Verification items for the finished model (mm, model axes). Coordinates: 2 decimals unless noted, no trailing zeros. Loops run counter-clockwise (first coordinate to the right, second up) from the corner with the lowest first, then second, coordinate; pieces in that order, holes last. Notation, with made-up numbers: (23, -39) - (45, -39) arc R8 ccw to (45, -26) - close; hole circle Ø2 at (-8, 71.25). An arc over 180 degrees is marked (long way). One line per item, written item: value. Start each with the question number.
(1) Section check C-C (x = 388). Record the boundary of the cut face in (y, z) (3 decimals).
(2) Gauge pin test, flat ends, axial feed: P1, Ø12, axis at y = -497, z = 12.5, coming from the -X side; P2, Ø8, axis at y = -641.5, z = 17.5, coming from the -X side. Record the tip position at first contact, or that the pin passes through.
(3) Draft check along Z on faces 1 (the face through (-15, -110, 28.575)), 2 (the face through (-15.65, -882.386, 14.087)), 3 (the face through (-15, -110, 0)). Enter one of: +Z half, -Z half, draft (parallel to the pull), parting line (faces both ways), or undercut.
(4) Section check B-B (x = 73.5). Record the boundary of the cut face in (y, z) (3 decimals), plus the area to 3 significant figures.
(5) Section check D-D (x = -331.5). Record the boundary of the cut face in (y, z) (3 decimals).
(6) Section check A-A (z = 5.5). Record the boundary of the cut face in (x, y).
(7) Thickness scan on probe 1 along Y at (x, z) = (0, 12.25); probe 2 along X at (y, z) = (-188.5, 19.5); probe 3 along Y at (x, z) = (-6, 17.5). Record the ranges inside material, lowest first. Write a range as [from, to].
```python
from build123d import *

# Parameters (mm, degrees)
F1_DEPTH = 28.575


# Not quite as in the source:
# - a feature names something its author has since deleted; it is built from what else it names


with BuildPart() as f1:
    # F0 (on Top) → F1 (new body)
    with BuildSketch(Plane.XY):
        with BuildLine():
            ThreePointArc((-1037.5478672986, -524.8695620945), (-548.7202955818, -790.5538516378), (0, -882.4590952158))
            ThreePointArc((0, -882.4590952158), (548.7202955818, -790.5538516378), (1037.5478672986, -524.8695620945))
            ThreePointArc((1037.5478672986, -524.8695620945), (1059.0976915237, -498.2343056164), (1066.8, -464.8500839552))
            Line((1066.8, -464.8500839552), (1066.8, -44.2590952158))
            Line((1066.8, -44.2590952158), (1066.8, 641.5409047842))
            Line((1066.8, 641.5409047842), (-1066.8, 641.5409047842))
            Line((-1066.8, 641.5409047842), (-1066.8, -44.2590952158))
            Line((-1066.8, -44.2590952158), (-1066.8, -464.8500839552))
            ThreePointArc((-1066.8, -464.8500839552), (-1059.0976915237, -498.2343056164), (-1037.5478672986, -524.8695620945))
        make_face()
        Polygon((-139.7, -165.1), (0, -165.1), (139.7, -165.1), (139.7, -292.1), (0, -292.1), (-139.7, -292.1), align=None, mode=Mode.SUBTRACT)
        with BuildLine():
            ThreePointArc((0, -25.4), (-17.9605122421, 17.9605122421), (25.4, 0))
            ThreePointArc((25.4, 0), (17.9605122421, -17.9605122421), (0, -25.4))
        make_face(mode=Mode.SUBTRACT)
    extrude(amount=F1_DEPTH)


solid = f1.part
```
Responses:
1. outline: (-837.152, 0) - (641.541, 0) - (641.541, 28.575) - (-837.152, 28.575) - close
2. P1: stops at x = -1062.17
2. P2: stops at x = -874.66
3. face 1: +Z half
3. face 2: draft
3. face 3: -Z half
4. outline: (-880.854, 0) - (-292.1, 0) - (-292.1, 28.575) - (-880.854, 28.575) - close; (-165.1, 0) - (641.541, 0) - (641.541, 28.575) - (-165.1, 28.575) - close
4. area: 39,900 mm²
5. outline: (-849.509, 0) - (641.541, 0) - (641.541, 28.575) - (-849.509, 28.575) - close
6. outline: (-1066.8, -464.85) arc R76.2 ccw to (-1037.55, -524.87) arc R1684.02 ccw to (1037.55, -524.87) arc R76.2 ccw to (1066.8, -464.85) - (1066.8, 641.54) - (-1066.8, 641.54) - close; hole (-139.7, -292.1) - (139.7, -292.1) - (139.7, -165.1) - (-139.7, -165.1) - close; hole circle Ø50.8 at (0, 0)
7. probe 1: y = [-882.46, -292.1], [-165.1, -25.4], [25.4, 641.54]
7. probe 2: x = [-1066.8, -139.7], [139.7, 1066.8]
7. probe 3: y = [-882.45, -292.1], [-165.1, -24.68], [24.68, 641.54]
